Geometry: see drawing. Coordinates: mm, zero at the bounding-box minimum. Round coordinates to 2 decimals unless told otherwise and drop trailing zeros. Write each loop counter-clockwise with the first axis right and the second up, starting at its lowest first coordinate (ties: lowest second). Pieces come first, ordered by that corner, then holes.
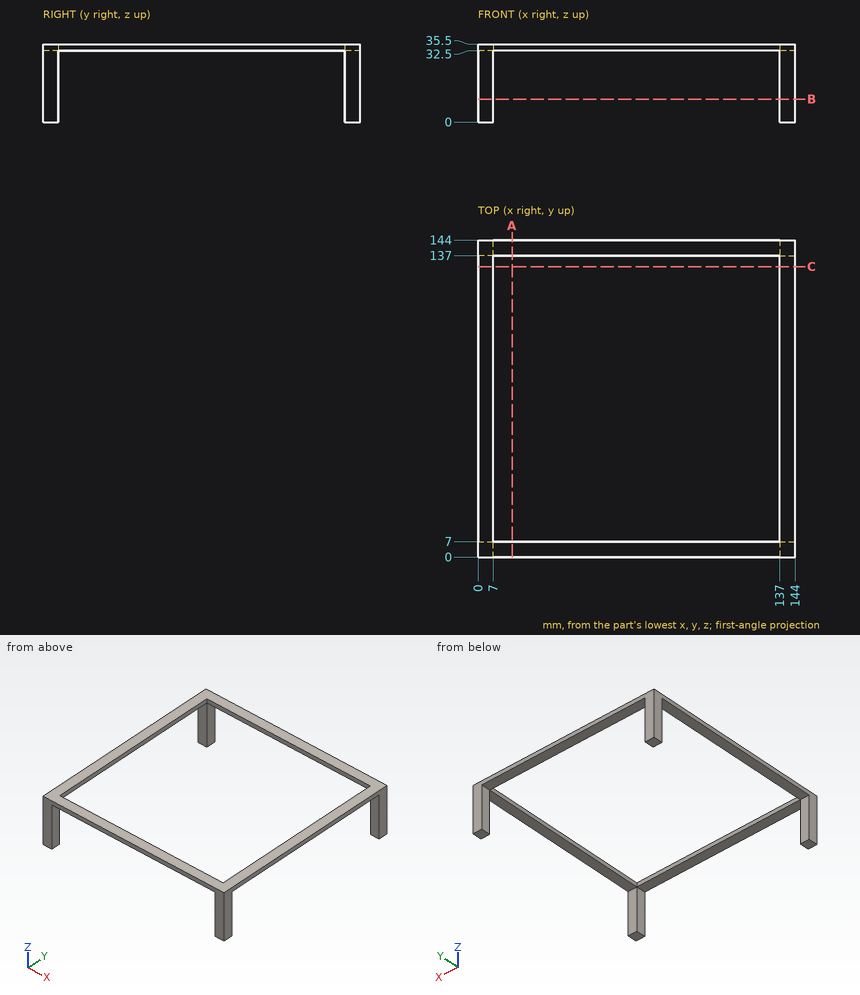
1) Material intervals for line 1 (Y direction, x = 138, z = 4.5); line 2 (Z direction, x = 39.5, y = 138), sorted ascending.
Taken from the geometry:
line 1: y = 0 to 7, 137 to 144
line 2: z = 32.5 to 35.5
2) Contact query for flat-ended pins moving along their axis: P1, Ø5.5, axis at x = 139.5, y = 86.5, coming from the -Z side; P2, Ø8, axis at y = 45.5, z = 27, coming from the -X side. Output: stop coordinate, or through.
Taken from the geometry:
P1: stops at z = 32.5
P2: passes through
3) Section query B-B on z = 10.5. Return the cut outline in (x, y).
Taken from the geometry:
outline: (0, 0) - (7, 0) - (7, 7) - (0, 7) - close; (0, 137) - (7, 137) - (7, 144) - (0, 144) - close; (137, 0) - (144, 0) - (144, 7) - (137, 7) - close; (137, 137) - (144, 137) - (144, 144) - (137, 144) - close
4) Section query A-A on x = 15.5. Return the cut outline in (y, z).
Taken from the geometry:
outline: (0, 32.5) - (7, 32.5) - (7, 35.5) - (0, 35.5) - close; (137, 32.5) - (144, 32.5) - (144, 35.5) - (137, 35.5) - close
